Input: part model. Units: mm. Frame: model coordinates. A direction names the side the tool comes from. Give positions to 0.01 mm unless a question says otherwise; leave off trailing zeros. Write each loop counter-clockwise with the first axis right and the second up, starting at its lowest first coordinate (ties: lowest second). Pieces come first, ordered by that corner, then holes. Notation, with made-up numbers: (23.25, -0.5) - (57.25, -0.5) arc R4 ccw to (57.25, 6.5) - close; hole circle Ø11 at (-15, -27). An arc over 180 degrees is marked (long way). Use a Markdown table: item, result. Add a question column.
1. Section query B-B, the plane z = 3. Return loops of the section in (x, y), plus the area to 3 significant figures.
2. Mould query, pull axis Z, two halves, no side actions, for faces 6 (the flat face through (50, 21, 0)), 7 (the flat face through (12, 26, -25)), 8 (the flat face through (26.515, 33.411, 0.245)). Classes: released by +Z, released by -Z, zero draft, split by the parting line, or undercut.
3. Material intervals for probe 1 along Z at (x, y) = (11, 39.5); probe 2 along Z at (x, y) = (39, 37); probe 3 along Z at (x, y) = (36, 8.5), sorted ascending.
4. Section query A-A, the plane y = 49. Return loops of the section in (x, z), plus the area to 3 significant figures.
5. Section query C-C, the plane z = 30.5. Return loops of the section in (x, y), plus the area to 3 significant figures.
6. Pin query (flat end, axial travel): pin 1 (10 mm diameter, centred on x = 0.5, y = 37, fed in from +Z); pin 2 (4 mm diameter, centred on x = 20.5, z = 27.5, fed in from +Y); pin 3 (1.5 mm diameter, centred on x = -34.5, z = 16, fed in from +Y). Return the tip coordinate at first contact, or that it passes through.
7. Set-up query: faces 1 (the flat face through (40, 41, -17.5)), 2 (the flat face through (-50, 1, -27)), 3 (the flat face through (50, 60, 24)), 4 (the flat face through (12, 26, 25)), 5 (the flat face through (-14.042, 21.972, -22.254)). Return all of +Z, -Z, +X, -X, +Y, -Y with unobstructed straight access to the full face (end or side cutting, diameter ignored); none if empty.
```python
from build123d import *

# Parameters (mm, degrees)
SKETCH3_W               = 100
SKETCH3_H               = 70
BOSS_EXTRUDE2_DEPTH     = 2
BOSS_EXTRUDE3_DEPTH     = 25
SKETCH7_W               = 35
SKETCH7_H               = 35
CUT_EXTRUDE3_DEPTH      = 20
CUT_EXTRUDE1_DEPTH      = 125.171613843
CUT_EXTRUDE1_DEPTH_BACK = 80
SKETCH8_W               = 44
SKETCH8_H               = 7.480636053
CUT_EXTRUDE4_DEPTH      = 101.661811193
SKETCH9_W               = 3
SKETCH9_H               = 2
CUT_EXTRUDE5_DEPTH      = 2


with BuildPart() as part:
    # Sketch3 → Boss-Extrude2 (new body)
    with BuildSketch(Plane(origin=(0, 0, 0), x_dir=(1, 0, 0), z_dir=(0, 1, 0))):
        Rectangle(SKETCH3_W, SKETCH3_H)
    extrude(amount=BOSS_EXTRUDE2_DEPTH)

    # Sketch4 → Boss-Extrude3 (add, symmetric)
    with BuildSketch(Plane.XY):
        Polygon((50, 62.735026919), (50, 2), (-50, 2), (-50, 5), align=None)
    extrude(amount=BOSS_EXTRUDE3_DEPTH, both=True)

    # Sketch7 → Cut-Extrude3 (cut)
    with BuildSketch(Plane(origin=(-14.665063509, 25.400635095, 0), x_dir=(0.8660254037844414, 0.49999999999999517, 0), z_dir=(-0.49999999999999517, 0.8660254037844414, 0))):
        with Locations((57.168783649, 0)):
            Rectangle(SKETCH7_W, SKETCH7_H)
    extrude(amount=-CUT_EXTRUDE3_DEPTH, mode=Mode.SUBTRACT)

    # Sketch5 → Cut-Extrude1 (cut, two sides: drawn at the far end of the back side and taken through both)
    with BuildSketch(Plane(origin=(-35.334936491, -20.400635095, 0), x_dir=(0, 0, -1), z_dir=(-0.8660254037844416, -0.4999999999999951, 0)).offset(-CUT_EXTRUDE1_DEPTH_BACK)):
        with BuildLine():
            Line((-22.5, -21.849490966), (22.5, -21.849490966))
            ThreePointArc((22.5, -21.849490966), (24.6, -23.949490966), (22.5, -26.049490966))
            Line((22.5, -26.049490966), (22, -26.049490966))
            Line((22, -26.049490966), (22, -29.330127019))
            Line((22, -29.330127019), (-22, -29.330127019))
            Line((-22, -29.330127019), (-22, -26.049490966))
            Line((-22, -26.049490966), (-22.5, -26.049490966))
            ThreePointArc((-22.5, -26.049490966), (-24.6, -23.949490966), (-22.5, -21.849490966))
        make_face()
    extrude(amount=CUT_EXTRUDE1_DEPTH + CUT_EXTRUDE1_DEPTH_BACK, mode=Mode.SUBTRACT)

    # Sketch8 → Cut-Extrude4 (cut, through all)
    with BuildSketch(Plane(origin=(33.947095812, 19.599364905, 0), x_dir=(0, 0, 1), z_dir=(-0.8660254037844414, -0.49999999999999517, 0))):
        with Locations((0, 25.589808993)):
            Rectangle(SKETCH8_W, SKETCH8_H)
    extrude(amount=-CUT_EXTRUDE4_DEPTH, mode=Mode.SUBTRACT)

    # Sketch9 → Cut-Extrude5 (cut)
    with BuildSketch(Plane(origin=(50, 0, 0), x_dir=(0, 0, -1), z_dir=(1, 0, 0))):
        with Locations((-23.5, 57.235026919)):
            Rectangle(SKETCH9_W, SKETCH9_H)
        with Locations((23.5, 57.235026919)):
            Rectangle(SKETCH9_W, SKETCH9_H)
    extrude(amount=-CUT_EXTRUDE5_DEPTH, mode=Mode.SUBTRACT)


solid = part.part
```
Result sheet:
| question | item | result |
|---|---|---|
| 1 | outline | (-43.7, 0) - (50, 0) - (50, 39.64) - (29.69, 27.91) - (23.43, 38.76) - close |
| 1 | area | 2,200 mm² |
| 2 | face 6 | zero draft |
| 2 | face 7 | released by -Z |
| 2 | face 8 | undercut |
| 3 | probe 1 | z = -25 to -22, 22 to 25 |
| 3 | probe 2 | z = -25 to -17.5, 17.5 to 25 |
| 3 | probe 3 | z = -25 to 25 |
| 4 | outline | (26.21, -25) - (50, -25) - (50, -17.5) - (41.17, -17.5) - (41.17, -22) - (26.21, -22) - close; (26.21, 22) - (41.17, 22) - (41.17, 17.5) - (50, 17.5) - (50, 25) - (26.21, 25) - close |
| 4 | area | 222 mm² |
| 5 | outline | (-50, 0) - (50, 0) - (50, 2) - (-50, 2) - close |
| 5 | area | 200 mm² |
| 6 | pin 1 | stops at z = 25 |
| 6 | pin 2 | stops at y = 2 |
| 6 | pin 3 | stops at y = 5.74 |
| 7 | face 1 | +Y |
| 7 | face 2 | +Z, -Z, -X, +Y, -Y |
| 7 | face 3 | +Z, -Z, +X, +Y, -Y |
| 7 | face 4 | +Z, +X, -X, +Y |
| 7 | face 5 | none |
